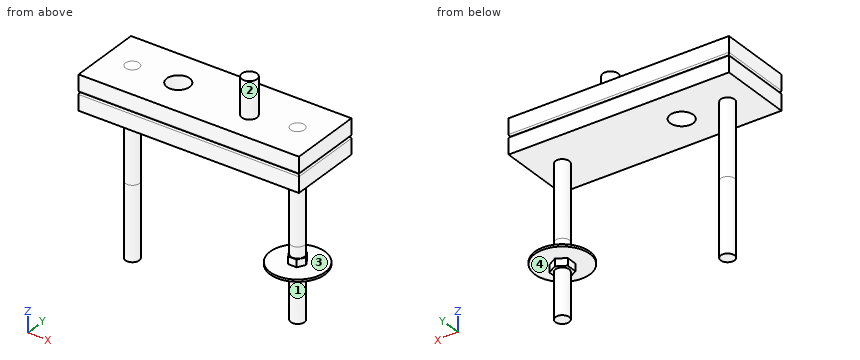
from build123d import *

# Parameters (mm, degrees)
F0_W      = 152.4
F0_H      = 50.8
F0_R      = 4.7625
F0_R_2    = 7.9375
F1_DEPTH  = 11.9888
F2_R      = 1.27
F4_R      = 4.7625
F5_DEPTH  = 76.2
F6_R      = 4.7625
F7_DEPTH  = 50.8
F9_R      = 19.05
F10_DEPTH = 1.524
F12_DEPTH = 5.08
F14_DEPTH = 5.08
F15_R     = 5.2764150672
F16_DEPTH = 25.4


with BuildPart() as f1:
    # F0 (on Top) → F1 (new body)
    with BuildSketch(Plane.XY):
        Rectangle(F0_W, F0_H)
        with Locations((-57.15, 0)):
            Circle(F0_R, mode=Mode.SUBTRACT)
        with Locations((-25.4, 0)):
            Circle(F0_R_2, mode=Mode.SUBTRACT)
        with Locations((57.15, 0)):
            Circle(F0_R, mode=Mode.SUBTRACT)
    extrude(amount=F1_DEPTH)

    # F2
    f2_edges = [f1.edges().sort_by_distance(p)[0] for p in [
        (0, 25.4, 0),
        (-76.2, 0, 0),
        (0, -25.4, 0),
        (76.2, 0, 0),
    ]]
    fillet(f2_edges, radius=F2_R)

    # F3: F1 across plane


with BuildPart() as f1_1:
    add(f1.part)
    add(f1.part.mirror(Plane.XY))

    # F4 (on face) → F5 (join)
    with BuildSketch(Plane.XY.offset(11.9888)):
        with Locations((-57.15, 0)):
            Circle(F4_R)
        with Locations((57.15, 0)):
            Circle(F4_R)
    extrude(amount=-F5_DEPTH)

    # F6 (on face) → F7 (join)
    with BuildSketch(Plane(origin=(0, 0, -64.2112), x_dir=(1, 0, 0), z_dir=(0, 0, -1))):
        with Locations((57.15, 0)):
            Circle(F6_R)
        with Locations((-57.15, 0)):
            Circle(F6_R)
    extrude(amount=F7_DEPTH)

    # F9 (on offset) → F10 (join)
    with BuildSketch(Plane(origin=(0, 0, -76.9112), x_dir=(1, 0, 0), z_dir=(0, 0, -1))):
        with Locations((57.15, 0)):
            Circle(F9_R)
    extrude(amount=F10_DEPTH)

    # F11 (on face) → F12 (join)
    with BuildSketch(Plane(origin=(0, 0, -78.4352), x_dir=(1, 0, 0), z_dir=(0, 0, -1))):
        Polygon((63.5, 3.6661742094), (57.15, 7.3323484187), (50.8, 3.6661742094), (50.8, -3.6661742094), (57.15, -7.3323484187), (63.5, -3.6661742094), align=None)
    extrude(amount=F12_DEPTH)

    # F13 (on face) → F14 (join)
    with BuildSketch(Plane.XY.offset(-76.9112)):
        Polygon((60.0829393675, -5.08), (63.015878735, 0), (60.0829393675, 5.08), (54.2170606325, 5.08), (51.284121265, 0), (54.2170606325, -5.08), align=None)
    extrude(amount=F14_DEPTH)

    # F15 (on face) → F16 (join)
    with BuildSketch(Plane.XY.offset(11.9888)):
        with Locations((27.2953044623, -4.8705367371)):
            Circle(F15_R)
    extrude(amount=F16_DEPTH)


solid = f1_1.part
Could you check a few things on this model? Use its own coordinates, in mm. Face numbers are marked on the shaded views. A direction names the side the tool comes from. Round coordinates to 2 decimals unless told otherwise and drop trailing zeros. Order: outer loops, then holes, each group sorted by start corner. A loop starts at its lowest first (then second) coordinate and runs counter-clockwise, first axis right, second up.
Q1. Imagine slicing it at A-A, the plane z = 8. List the corners of the cut face in (x, y) for me (1 decimal).
Geometry says:
outline: (-76.2, -25.4) - (76.2, -25.4) - (76.2, 25.4) - (-76.2, 25.4) - close; hole circle Ø15.9 at (-25.4, 0)
Q2. I'm going to push flat-ended pins straight in: P1, Ø1.5, axis at x = 0.5, y = -0.5, coming from the -Z side; P2, Ø1.5, axis at x = 57, z = -73.5, coming from the -Y side; P3, Ø3, axis at x = 55, y = 2.5, coming from the +Z side. Where does each tip first touch, or does it pass through?
Geometry says:
P1: stops at z = -11.99
P2: stops at y = -5.08
P3: stops at z = 11.99
Q3. Please list where these lines run through material, in increasing order: probe 1 along Y at (x, z) = (-25.4, -5); probe 2 along Z at (x, y) = (37, 7.5); probe 3 along Z at (x, y) = (52, -5.5).
Geometry says:
probe 1: y = -25.4 to -7.94, 7.94 to 25.4
probe 2: z = -11.99 to 11.99
probe 3: z = -78.44 to -76.91, -11.99 to 11.99
Q4. Imagine slicing it at C-C, the plane x = -22.5. List the corners of the cut face in (y, z) for me, then the cut area to 3 significant figures.
Geometry says:
outline: (-25.4, -11.99) - (-7.39, -11.99) - (-7.39, 11.99) - (-25.4, 11.99) - (-25.4, 1.27) arc R1.27 ccw to (-24.13, 0) arc R1.27 ccw to (-25.4, -1.27) - close; (7.39, -11.99) - (25.4, -11.99) - (25.4, -1.27) arc R1.27 ccw to (24.13, 0) arc R1.27 ccw to (25.4, 1.27) - (25.4, 11.99) - (7.39, 11.99) - close
area: 862 mm2
Q5. Imagine slicing it at D-D, the plane y = -21. List the corners of the cut face in (x, z) for me, then the cut area to 3 significant figures.
Geometry says:
outline: (-76.2, -11.99) - (76.2, -11.99) - (76.2, -1.27) arc R1.27 ccw to (74.93, 0) arc R1.27 ccw to (76.2, 1.27) - (76.2, 11.99) - (-76.2, 11.99) - (-76.2, 1.27) arc R1.27 ccw to (-74.93, 0) arc R1.27 ccw to (-76.2, -1.27) - close
area: 3,650 mm2
Q6. Imagine slicing it at B-B, the plane x = -57.15. List the corners of the cut face in (y, z) for me.
Geometry says:
outline: (-25.4, -11.99) - (-4.76, -11.99) - (-4.76, -115.01) - (4.76, -115.01) - (4.76, -11.99) - (25.4, -11.99) - (25.4, -1.27) arc R1.27 ccw to (24.13, 0) arc R1.27 ccw to (25.4, 1.27) - (25.4, 11.99) - (-25.4, 11.99) - (-25.4, 1.27) arc R1.27 ccw to (-24.13, 0) arc R1.27 ccw to (-25.4, -1.27) - close
Q7. Which directions (+Z, -Z, +X, -X, +Y, -Y) give clear straight access to the entire face, cutting with the end or side of a thin tool? Please do the marked faces 3 and 4.
Geometry says:
face 3: none
face 4: -Z
Q8. Thinking about a two-plate mould opening in X: for the marked faces 1 and 2, which applies, released by +X, released by -X, zero draft, split by the parting line, or undercut?
Geometry says:
face 1: undercut
face 2: split by the parting line
